Here's how the part is built. I have some questions about the finished solid (model axes, mm). Face numbers are marked on the shaded views. A direction names the side the tool comes from. Give positions to 0.01 mm unless a question says otherwise; leave off trailing zeros. Order: outer loops, then holes, each group sorted by start corner. A loop starts at its lowest first (then second) coordinate and runs counter-clockwise, first axis right, second up.
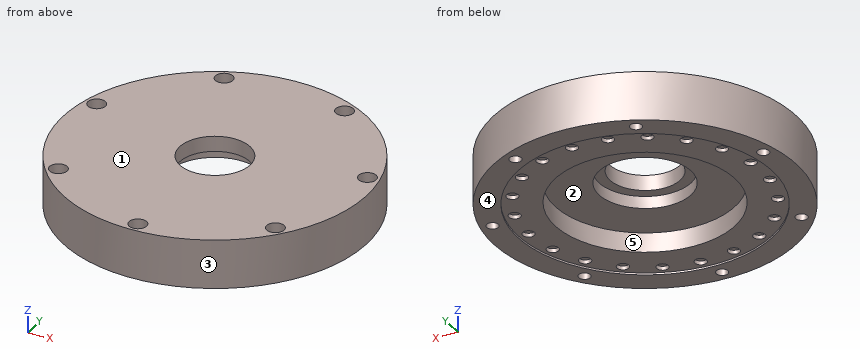
Autodesk Inventor part; units mm, degrees
ref_plane "YZ Plane" through (0, 0, 0) normal (1, 0, 0) x (0, 1, 0)
ref_plane "XZ Plane" through (0, 0, 0) normal (0, 1, 0) x (-1, 0, 0)
ref_plane "XY Plane" through (0, 0, 0) normal (0, 0, 1) x (1, 0, 0)
sketch "Sketch1" plane through (0, 0, 0) normal (0, 0, 1) x (1, 0, 0)
  circle A0 centre (0, 0) radius 77.5
  dimension "d0" = 155
extrude "Extrusion1" add sketch "Sketch1" along normal blind 25
sketch "Sketch2" plane through (0, 0, 0) normal (0, 0, -1) x (-1, 0, 0)
  circle A0 centre (-60, 0) radius 3
  circle A1 centre (0, 0) radius 60 construction
  circle A2 centre (-57.3344, -17.6853) radius 3
  circle A3 centre (-49.5743, -33.7992) radius 3
  circle A4 centre (-37.4094, -46.9099) radius 3
  circle A5 centre (-21.9205, -55.8524) radius 3
  circle A6 centre (-4.4838, -59.8322) radius 3
  circle A7 centre (13.3513, -58.4957) radius 3
  circle A8 centre (30, -51.9615) radius 3
  circle A9 centre (43.9831, -40.8104) radius 3
  circle A10 centre (54.0581, -26.033) radius 3
  circle A11 centre (59.3298, -8.9425) radius 3
  circle A12 centre (59.3298, 8.9425) radius 3
  circle A13 centre (54.0581, 26.033) radius 3
  circle A14 centre (43.9831, 40.8104) radius 3
  circle A15 centre (30, 51.9615) radius 3
  circle A16 centre (13.3513, 58.4957) radius 3
  circle A17 centre (-4.4838, 59.8322) radius 3
  circle A18 centre (-21.9205, 55.8524) radius 3
  circle A19 centre (-37.4094, 46.9099) radius 3
  circle A20 centre (-49.5743, 33.7992) radius 3
  circle A21 centre (-57.3344, 17.6853) radius 3
  dimension "d4" = 120
  dimension "d3" = 6
  dimension "d7" = 360
extrude "Extrusion2" cut sketch "Sketch2" against normal blind 3
sketch "Sketch3" plane through (0, 0, 25) normal (0, 0, 1) x (1, 0, 0)
  circle A0 centre (0, 0) radius 18
  dimension "d11" = 36
extrude "Extrusion3" cut sketch "Sketch3" against normal through all
sketch "Sketch4" plane through (0, 0, 0) normal (0, 0, -1) x (-1, 0, 0)
  circle A0 centre (0, 0) radius 46
  dimension "d14" = 92
extrude "Extrusion4" cut sketch "Sketch4" against normal blind 11
sketch "Sketch5" plane through (0, 0, 25) normal (0, 0, 1) x (1, 0, 0)
  circle A0 centre (0, 0) radius 71.5 construction
  point P0 (-0.0461, -71.5)
  dimension "d24" = 143
hole "Hole" at (-0.0461, -71.5, 25) direction (0, 0, -1) diameter 6 end through all counterbore diameter 9 counterbore depth 5.5
pattern_circular "Circular Pattern1" count 7 over 360 about axis through (0, 0, -10) along (0, 0, 1) of "Hole"
sketch "Sketch6" plane through (0, 0, 0) normal (0, 0, -1) x (-1, 0, 0)
  circle A0 centre (0, 0) radius 65
  dimension "d28" = 130
extrude "Extrusion5" cut sketch "Sketch6" against normal blind 1
sketch "Sketch7" plane through (0, 0, 11) normal (0, 0, -1) x (-1, 0, 0)
  circle A0 centre (0, 0) radius 23.5
  dimension "d31" = 47
extrude "Extrusion6" cut sketch "Sketch7" against normal blind 6.2
properties part number "Lid Case"
Q1. If we section it at B-B on x = -30: List the corners of the cut face in (y, z) for me, plus the area to 3 significant figures.
Filled sheet:
outline: (-71.46, 0) - (-57.66, 0) - (-57.66, 1) - (-54.96, 1) - (-54.96, 3) - (-48.96, 3) - (-48.96, 1) - (-34.87, 1) - (-34.87, 11) - (34.87, 11) - (34.87, 1) - (48.96, 1) - (48.96, 3) - (54.96, 3) - (54.96, 1) - (57.66, 1) - (57.66, 0) - (61.6, 0) - (61.6, 19.5) - (60.05, 19.5) - (60.05, 25) - (-71.46, 25) - close; (67.27, 0) - (71.46, 0) - (71.46, 25) - (68.83, 25) - (68.83, 19.5) - (67.27, 19.5) - close
area: 2,580 mm2
Q2. If we section it at D-D on x = 30.5: List the corners of the cut face in (y, z) for me, plus the area to 3 significant figures.
Filled sheet:
outline: (-71.25, 0) - (-57.4, 0) - (-57.4, 1) - (-34.43, 1) - (-34.43, 11) - (34.43, 11) - (34.43, 1) - (57.4, 1) - (57.4, 0) - (61.45, 0) - (61.45, 19.5) - (59.93, 19.5) - (59.93, 25) - (-71.25, 25) - close; (67.35, 0) - (71.25, 0) - (71.25, 25) - (68.86, 25) - (68.86, 19.5) - (67.35, 19.5) - close
area: 2,590 mm2
Q3. I'm going to push flat-ended pins straight in: P1, Ø3, axis at x = -60, y = -8, coming from the -Z side; P2, Ø6.5, axis at x = -30.5, y = 53.5, coming from the -Z side; P3, Ø1, axis at x = -41.5, z = 17.5, coming from the +Y side. Where does each tip first touch, or does it pass through?
Filled sheet:
P1: stops at z = 3
P2: stops at z = 1
P3: stops at y = 65.77
Q4. For the marked faces 4 and 5, which set-ups out of +Z, -Z, +X, -X, +Y, -Y let a thin tool reach every point of the face, with its end or its side?
Filled sheet:
face 4: -Z, +X, -X, +Y, -Y
face 5: -Z
Q5. I need wall thicknesses on L1, parallel to Y at x = 0, z = 3.5; L2, parallel to X at y = 65.5, z = 11.5 (3 decimals); L3, parallel to X at y = 58, z = 1.5. Which ranges of each line are inside material? Lowest first, please.
Filled sheet:
L1: y = -77.5 to -74.5, -68.5 to -46, 46 to 77.5
L2: x = -41.425 to -33.787, -28.175 to 28.273, 33.855 to 41.425
L3: x = -51.4 to -16.31, -10.39 to 2.11, 6.86 to 19.83, 24.02 to 51.4
Q6. If we section it at C-C on y = -71.5: List the corners of the cut face in (x, z) for me, plus the area to 3 significant figures.
Filled sheet:
outline: (-29.9, 0) - (-3.05, 0) - (-3.05, 19.5) - (-4.55, 19.5) - (-4.55, 25) - (-29.9, 25) - close; (2.95, 0) - (29.9, 0) - (29.9, 25) - (4.45, 25) - (4.45, 19.5) - (2.95, 19.5) - close
area: 1,330 mm2
Q7. Thinking about a two-plate mould opening in X: for the marked faces 1, 2 and 3, which applies, released by +X, released by -X, zero draft, split by the parting line, or undercut?
Filled sheet:
face 1: zero draft
face 2: undercut
face 3: split by the parting line
Q8. If we section it at A-A on y = 0: List the corners of the cut face in (x, z) for me.
Filled sheet:
outline: (-77.5, 0) - (-65, 0) - (-65, 1) - (-46, 1) - (-46, 11) - (-23.5, 11) - (-23.5, 17.2) - (-18, 17.2) - (-18, 25) - (-77.5, 25) - close; (18, 17.2) - (23.5, 17.2) - (23.5, 11) - (46, 11) - (46, 1) - (57, 1) - (57, 3) - (63, 3) - (63, 1) - (65, 1) - (65, 0) - (77.5, 0) - (77.5, 25) - (18, 25) - close
